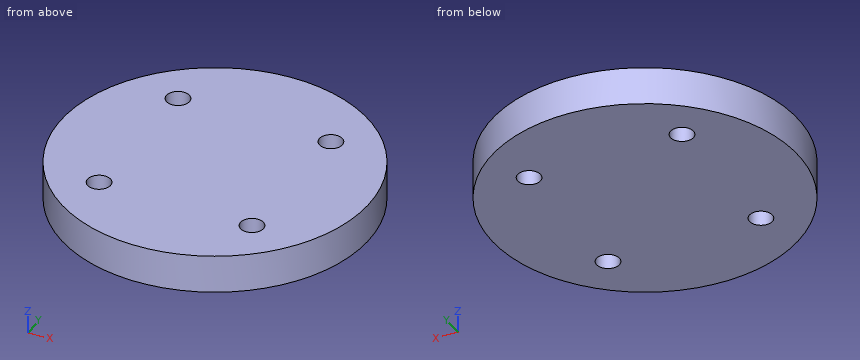
from build123d import *

# Parameters (mm, degrees)
SKETCH_1_R      = 20
SKETCH_1_R_2    = 1.5
EXTRUDE_1_DEPTH = 5


with BuildPart() as part:
    # 草圖1 → 填料-伸長1 (new body)
    with BuildSketch(Plane.XY):
        Circle(SKETCH_1_R)
        with Locations((-10, -10)):
            Circle(SKETCH_1_R_2, mode=Mode.SUBTRACT)
        with Locations(Location((-10, 10, 0), (0, 0, 180))):
            Circle(SKETCH_1_R_2, mode=Mode.SUBTRACT)
        with Locations((10, 10)):
            Circle(SKETCH_1_R_2, mode=Mode.SUBTRACT)
        with Locations(Location((10, -10, 0), (0, 0, 180))):
            Circle(SKETCH_1_R_2, mode=Mode.SUBTRACT)
    extrude(amount=EXTRUDE_1_DEPTH)


solid = part.part
Design review of the part built by this model. Coordinates are the model's own, in mm. Round coordinates to 2 decimals unless told otherwise and drop trailing zeros. Write each loop counter-clockwise with the first axis right and the second up, starting at its lowest first coordinate (ties: lowest second). Pieces come first, ordered by that corner, then holes. Notation, with made-up numbers: (-15.5, 72) - (27.5, 72) arc R34 ccw to (27.5, 108) - close; hole circle Ø4 at (10, 29.25). An arc over 180 degrees is marked (long way). Return JSON: item names as keys, results as strings. Group by question number.
Item 1: Insertion check: P1, Ø1.5, axis at y = 7, z = 1, coming from the -X side; P2, Ø1.8, axis at x = 10, y = -10, coming from the +Z side; P3, Ø3, axis at x = 6.5, z = 1, coming from the -Y side. Each pin has a flat end and moves straight along its axis. Give the tip position at first contact, or say it passes through.
Item 2: We need section A-A on x = 10. Write out the cut boundary in (y, z).
Item 3: For probe 1 along X at (y, z) = (-9, 2); probe 2 along X at (y, z) = (-0.5, 0.95); probe 3 along Y at (x, z) = (0, 0.7), list the stretches that pass through material, from the lowest coordinate up. Write a range as [from, to].
Item 4: We need section B-B on z = 1.2. Write out the cut boundary in (x, y).
Item 5: We need section D-D on y = -5. Write out the cut boundary in (x, z).
Model answer:
{
 "1": {"P1": "stops at x = -19", "P2": "passes through", "P3": "stops at y = -19.36"},
 "2": {"outline": "(-17.32, 0) - (-11.5, 0) - (-11.5, 5) - (-17.32, 5) - close; (-8.5, 0) - (8.5, 0) - (8.5, 5) - (-8.5, 5) - close; (11.5, 0) - (17.32, 0) - (17.32, 5) - (11.5, 5) - close"},
 "3": {"probe 1": "x = [-17.86, -11.12], [-8.88, 8.88], [11.12, 17.86]", "probe 2": "x = [-19.99, 19.99]", "probe 3": "y = [-20, 20]"},
 "4": {"outline": "circle Ø40 at (0, 0); hole circle Ø3 at (-10, -10); hole circle Ø3 at (-10, 10); hole circle Ø3 at (10, -10); hole circle Ø3 at (10, 10)"},
 "5": {"outline": "(-19.36, 0) - (19.36, 0) - (19.36, 5) - (-19.36, 5) - close"}
}
